CAD build for the part. Positions are in the model's coordinates, mm. A direction names the side the tool comes from. Coordinates: 2 decimals unless noted, no trailing zeros. Write each loop counter-clockwise with the first axis right and the second up, starting at its lowest first coordinate (ties: lowest second). Pieces come first, ordered by that corner, then holes. Notation, with made-up numbers: M 45.5,-8 L 65.5,-8 A16 cw 65.5,18 Z; hole C 25,-4 d3. An arc over 180 degrees is marked long. Answer as CSV lines item,"result". Start each with the question number.
```python
from build123d import *

# Parameters (mm, degrees)
SKETCH1_W           = 25.4
SKETCH1_H           = 111.125
BOSS_EXTRUDE1_DEPTH = 1.5
SKETCH2_W           = 3.175
SKETCH2_H           = 9.525
BOSS_EXTRUDE2_DEPTH = 3
CUT_EXTRUDE1_DEPTH  = 3
FILLET1_R           = 0.79375
SKETCH5_W           = 3
SKETCH5_H           = 6.35
BOSS_EXTRUDE3_DEPTH = 3


with BuildPart() as part:
    # Sketch1 → Boss-Extrude1 (new, symmetric)
    with BuildSketch(Plane(origin=(0, 34.29, 0), x_dir=(1, 0, 0), z_dir=(0, 1, 0))):
        with Locations((0, 120.65)):
            Rectangle(SKETCH1_W, SKETCH1_H)
    extrude(amount=BOSS_EXTRUDE1_DEPTH, both=True)

    # Sketch2 → Boss-Extrude2 (add)
    with BuildSketch(Plane(origin=(0, 35.79, 0), x_dir=(1, 0, 0), z_dir=(0, 1, 0))):
        with Locations((14.2875, 171.45)):
            Rectangle(SKETCH2_W, SKETCH2_H)
        with Locations((-14.2875, 171.45)):
            Rectangle(SKETCH2_W, SKETCH2_H)
        with Locations((14.2875, 120.65)):
            Rectangle(SKETCH2_W, SKETCH2_H)
        with Locations((-14.2875, 120.65)):
            Rectangle(SKETCH2_W, SKETCH2_H)
        with Locations((14.2875, 69.85)):
            Rectangle(SKETCH2_W, SKETCH2_H)
        with Locations((-14.2875, 69.85)):
            Rectangle(SKETCH2_W, SKETCH2_H)
    extrude(amount=-BOSS_EXTRUDE2_DEPTH)

    # Sketch4 → Cut-Extrude1 (cut)
    with BuildSketch(Plane(origin=(0, 35.79, 0), x_dir=(1, 0, 0), z_dir=(0, 1, 0))):
        Polygon((7.83579899, 173.0375), (-9.525, 173.0375), (-9.525, 125.295302777), align=None)
        Polygon((9.525, 122.2375), (9.525, 168.392197223), (-7.258526263, 122.2375), align=None)
        Polygon((9.525, 119.0625), (-7.258526263, 119.0625), (9.525, 72.907802777), align=None)
        Polygon((7.83579899, 68.2625), (-9.525, 116.004697223), (-9.525, 68.2625), align=None)
    extrude(amount=-CUT_EXTRUDE1_DEPTH, mode=Mode.SUBTRACT)

    # Fillet1
    fillet1_edges = [part.edges().sort_by_distance(p)[0] for p in [
        (-7.258526263, 34.29, -122.2375),
        (9.525, 34.29, -168.392197223),
        (9.525, 34.29, -122.2375),
        (9.525, 34.29, -72.907802777),
        (-7.258526263, 34.29, -119.0625),
        (9.525, 34.29, -119.0625),
        (7.83579899, 34.29, -68.2625),
        (-9.525, 34.29, -68.2625),
        (-9.525, 34.29, -116.004697223),
        (-9.525, 34.29, -125.295302777),
        (-9.525, 34.29, -173.0375),
        (7.83579899, 34.29, -173.0375),
        (15.875, 34.29, -65.0875),
        (15.875, 34.29, -74.6125),
        (12.7, 34.29, -74.6125),
        (-12.7, 34.29, -115.8875),
        (-12.7, 34.29, -125.4125),
        (-15.875, 34.29, -125.4125),
        (-15.875, 34.29, -115.8875),
        (15.875, 34.29, -115.8875),
        (15.875, 34.29, -125.4125),
        (12.7, 34.29, -125.4125),
        (12.7, 34.29, -115.8875),
        (-12.7, 34.29, -166.6875),
        (-15.875, 34.29, -176.2125),
        (-15.875, 34.29, -166.6875),
        (-12.7, 34.29, -74.6125),
        (-15.875, 34.29, -74.6125),
        (-15.875, 34.29, -65.0875),
        (15.875, 34.29, -166.6875),
        (15.875, 34.29, -176.2125),
        (12.7, 34.29, -166.6875),
    ]]
    fillet(fillet1_edges, radius=FILLET1_R)

    # Sketch5 → Boss-Extrude3 (add)
    with BuildSketch(Plane(origin=(0, 35.79, 0), x_dir=(1, 0, 0), z_dir=(0, 1, 0))):
        with Locations((17.375, 171.45)):
            Rectangle(SKETCH5_W, SKETCH5_H)
        with Locations((-17.375, 171.45)):
            Rectangle(SKETCH5_W, SKETCH5_H)
        with Locations((17.375, 120.65)):
            Rectangle(SKETCH5_W, SKETCH5_H)
        with Locations((-17.375, 120.65)):
            Rectangle(SKETCH5_W, SKETCH5_H)
        with Locations((17.375, 69.85)):
            Rectangle(SKETCH5_W, SKETCH5_H)
        with Locations((-17.375, 69.85)):
            Rectangle(SKETCH5_W, SKETCH5_H)
    extrude(amount=-BOSS_EXTRUDE3_DEPTH)


solid = part.part
```
1) Band-saw the part on B-B, the plane z = -81. List the corners of the cut face in (x, y) (3 decimals), plus the area to 3 significant figures.
2) Pin check, flat tips, straight feed: P1, Ø1.5, axis at y = 33.5, z = -159.5, coming from the +X side; P2, Ø0.6, axis at y = 34.5, z = -73.5, coming from the -X side (3 decimals); P3, Ø1.5, axis at y = 34, z = -100.5, coming from the -X side. Stop position of each tip, or through.
3) Tool access for faces 4 (the flat face through (-9.525, 34, -91)), 5 (the flat face through (-17, 34, -123.825)), 6 (the flat face through (17, 34, -117.475)): list every direction of +Z, -Z, +X, -X, +Y, -Y with a clear straight run to the whole face (end or side of a thin tool).
4) Band-saw the part on C-C, the plane y = 35. State how many separate pieces and enclosed holes the cut face has, plus the area to 3 significant figures.
5) Probe L1, parallel to Z at x = -15, y = 33.25; L2, parallel to Z at x = 17, y = 34 (3 decimals); L3, parallel to X at y = 35.4, z = -141 (3 decimals). List the from-to ranges inside material, lowest first. Write a range as [from, to].
6) Band-saw the part on A-A, the plane x = -4.5. List the corners of the cut face in (y, z), plus the area to 3 significant figures.
7) Two-plate mould, pull along Z, no slides. Class faces 1 (the flat face through (17, 34, -123.825)), 2 (the flat face through (-0.376, 34.311, -150.454)), 3 (the flat face through (-18.875, 34, -70)): pulls with the +Z half, pulls with the -Z half, needs draft (parallel to the pull), parting line crosses it, or undercut.
Result sheet:
1,outline,"M -12.7,32.79 L -9.525,32.79 L -9.525,35.79 L -12.7,35.79 Z; M 3.204,32.79 L 6.582,32.79 L 6.582,35.79 L 3.204,35.79 Z; M 9.525,32.79 L 12.7,32.79 L 12.7,35.79 L 9.525,35.79 Z"
1,area,"29.2 mm²"
2,P1,"stops at x = 12.7"
2,P2,"stops at x = -15.875"
2,P3,"stops at x = -12.7"
3,face 4,"+Y, -Y"
3,face 5,"-X, +Y, -Y"
3,face 6,"+X, +Y, -Y"
4,separate pieces,"1"
4,enclosed holes,"4"
4,area,"1,530 mm²"
5,L1,"z = [-176.21, -166.69], [-125.41, -115.89], [-74.61, -65.09]"
5,L2,"z = [-174.625, -168.275], [-123.825, -117.475], [-73.025, -66.675]"
5,L3,"x = [-12.7, -9.525], [-3.814, -0.436], [9.525, 12.7]"
6,outline,"M 32.79,-176.21 L 35.79,-176.21 L 35.79,-173.04 L 32.79,-173.04 Z; M 32.79,-139.11 L 35.79,-139.11 L 35.79,-129.82 L 32.79,-129.82 Z; M 32.79,-122.24 L 35.79,-122.24 L 35.79,-119.06 L 32.79,-119.06 Z; M 32.79,-111.48 L 35.79,-111.48 L 35.79,-102.19 L 32.79,-102.19 Z; M 32.79,-68.26 L 35.79,-68.26 L 35.79,-65.09 L 32.79,-65.09 Z"
6,area,"84.3 mm²"
7,face 1,"undercut"
7,face 2,"undercut"
7,face 3,"needs draft"
